For this review, take the finished solid that the model builds, in its own axes (mm). A direction names the side the tool comes from. Give positions to 0.01 mm unless a question says otherwise; leave off trailing zeros. Loops run counter-clockwise (first coordinate to the right, second up) from the corner with the lowest first, then second, coordinate; pieces in that order, holes last. Notation, with made-up numbers: (0, 89) -> (23, 89) arc R19 cw to (23, 117) -> close; hole circle Ø7 at (16, 85.5). An arc over 180 degrees is marked (long way). Answer as CSV lines item,"result". Start each with the question number.
Item 1: Add section A-A on x = -47. State the section outline as (y, z) points, plus the area to 3 significant figures.
Item 2: Add section D-D on y = 225. State the section outline as (x, z) points.
Item 3: For L1, parallel to X at y = 184, z = -42; L2, parallel to Z at x = -282.3, y = 65; L3, parallel to Y at x = -283.3, z = -10, list the stretches that pass through material, from the lowest coordinate up. Write a range as from..to.
Item 4: Clearance check with flat-ended pins moving along their axes: P1, Ø12, axis at x = -95.5, y = 62, coming from the +Z side; P2, Ø8, axis at x = -248, y = 187.5, coming from the -Z side (3 decimals); P3, Ø8, axis at x = -152.5, z = 28.5, coming from the +Y side. State where each tip first meets the part, or that it passes through.
Item 5: Machinability: for faces 1 (the face through (-142.03, 195.48, -14.85)), 2 (the face through (-142, 44, 50)), 3 (the face through (-138, 111.5, -110.4)), which of the approach directions +Z, -Z, +X, -X, +Y, -Y give a long, thin tool a straight path to every point of the face, cutting with its end or side? Answer none if there is none.
Item 6: Add section C-C on z = -55.5. State the section outline as (x, y) points.
Item 7: Add section B-B on y = 132.5. State the section outline as (x, z) points, plus the area to 3 significant figures.
Item 8: The part is to be moulded in two halves that separate along Z. For faces 4 (the face through (-280, 133, -34)), 5 (the face through (-142.03, 43.014, 52.449)), 6 (the face through (5, 151, -34)), say which applies: +Z half, -Z half, draft (parallel to the pull), parting line (faces both ways), or undercut.
Autodesk Inventor part; units mm, degrees
ref_plane "YZ Plane" through (0, 0, 0) normal (1, 0, 0) x (0, 1, 0)
ref_plane "XZ Plane" through (0, 0, 0) normal (0, 1, 0) x (-1, 0, 0)
ref_plane "XY Plane" through (0, 0, 0) normal (0, 0, 1) x (1, 0, 0)
sketch "Sketch1" plane through (0, 0, 0) normal (1, 0, 0) x (0, 1, 0)
  line L0 (42.8643, -50) -> (204.4541, -208.7035)
  line L1 (0, 0) -> (0, -50)
  line L2 (124.4924, 56.8774) -> (295.5459, -115.955)
  line L3 (122.4584, 51.8246) -> (292.042, -119.5226)
  line L4 (50, -50) -> (207.9576, -205.1362)
  line L5 (295.5459, -115.955) -> (204.4541, -208.7035)
  circle A0 centre (250, -162.3292) radius 10
  circle A1 centre (250, -162.3292) radius 76
  line L6 (124.4924, 56.8774) -> (-148.62, 50)
  line L7 (50, 50) -> (122.4584, 51.8246)
  line L8 (0, 0) -> (0, -77.5)
  line L9 (-50, 50) -> (50, 50)
  line L10 (50, 50) -> (50, -50)
  line L11 (50, -50) -> (-50, -50)
  line L12 (-50, -50) -> (-50, 50)
  line L13 (-50, 50) -> (50, -50) construction
  line L14 (50, 50) -> (-50, -50) construction
  line L15 (37.5556, 50) -> (48.6277, 54.967)
  point P0 (22.0043, 0)
  point P1 (259.821, -86.9665)
  point P2 (268.4835, -88.6111)
  point P3 (176.3565, -181.1077)
  point P4 (174.6769, -172.4499)
  point P5 (242.9929, -169.4637)
  point P6 (257.0071, -155.1947)
  dimension "d6" = 5
  dimension "d7" = 5
  dimension "d8" = 90
  dimension "d9" = 130
  dimension "d11" = 50
  dimension "d14" = 20
  dimension "d16" = 152
  dimension "d17" = 250
  dimension "d18" = 5
  dimension "d24" = 77.5
  dimension "d26" = 264
  dimension "d29" = 100
  dimension "d30" = 100
extrude "Extrusion1" add sketch "Sketch1" against normal blind 280 contours L11 L4 A1 L0 | L9 L15 L6 L2 A1 L3 L7
extrude "Extrusion2" add sketch "Sketch1" along normal blind 5 contours L11 L4 A1 L0 | L10 L7 L3 A1 L4 | L9 L15 L6 L2 A1 L3 L7
ref_plane "Work Plane1" through (-140, 0, 0) normal (-1, 0, 0) x (0, 0, 1)
mirror "Mirror1" about plane through (-140, 0, 0) normal (-1, 0, 0) of "Extrusion2"
sketch "Sketch4" plane through (5, 0, 0) normal (1, 0, 0) x (0, 0, -1)
  arc A0 (88.6111, 268.4835) -> (181.1077, 176.3565) centre (162.3292, 250) ccw
  line L0 (88.6111, 268.4835) -> (-56.8774, 124.4924)
  line L1 (-56.8774, 124.4924) -> (-54.967, 48.6277)
  line L2 (-54.967, 48.6277) -> (-50, 37.5556)
  line L3 (-50, 37.5556) -> (-50, 50)
  line L4 (-50, 50) -> (50, 50)
  line L5 (50, 50) -> (50, 42.8643)
  line L6 (50, 42.8643) -> (181.1077, 176.3565)
  circle A1 centre (-10, 65) radius 1.5
  circle A2 centre (10, 65) radius 1.5
  line L7 (-10, 65) -> (10, 65)
  point P0 (0, 0)
  point P1 (0, 65)
  point P2 (0, 50)
  dimension "d31" = 15
  dimension "d32" = 3
  dimension "d33" = 3
  dimension "d34" = 20
extrude "Extrusion5" cut sketch "Sketch4" against normal through all contours A1 | A2
properties part number "CANALETA_GUIA" material "Steel, Mild, Welded"
Computed values:
1,outline,"(37.56, 50) -> (50, 50) -> (122.46, 51.82) -> (259.82, -86.97) arc R76 cw to (268.48, -88.61) -> (124.49, 56.88) -> (48.63, 54.97) -> close; (42.86, -50) -> (176.36, -181.11) arc R76 cw to (174.68, -172.45) -> (50, -50) -> close"
1,area,"2,300 mm²"
2,outline,"(-285, -90.56) -> (-280, -90.56) -> (-280, -51.78) -> (0, -51.78) -> (0, -90.56) -> (5, -90.56) -> (5, -44.68) -> (-285, -44.68) -> close"
3,L1,"-285..-280, 0..5"
3,L2,"-71.74..-11.5, -8.5..8.5, 11.5..55.38"
3,L3,"50..63.5, 66.5..190.68"
4,P1,"z = 55.45"
4,P2,"z = -17.935"
4,P3,"y = 156.54"
5,face 1,"+Z, +X, -X, +Y"
5,face 2,"+X, -X, -Y"
5,face 3,"none"
6,outline,"(-285, 48.46) -> (5, 48.46) -> (5, 235.71) -> (-285, 235.71) -> close; hole (-280, 55.6) -> (0, 55.6) -> (0, 228.68) -> (-280, 228.68) -> close"
7,outline,"(-285, -138.03) -> (5, -138.03) -> (5, 48.79) -> (-285, 48.79) -> close; hole (-280, -131.03) -> (0, -131.03) -> (0, 41.68) -> (-280, 41.68) -> close"
7,area,"5,820 mm²"
8,face 4,"undercut"
8,face 5,"+Z half"
8,face 6,"draft"
